Answer from the drawing. Dimensions are ordinates in mm from the lowest x, y and z of the part. Give positions to 0.01 mm unless a question says otherwise; leave off trailing zeros. Write each loop counter-clockwise with the first axis right and the second up, starting at its lowest first coordinate (ties: lowest second). Pieces come first, ordered by that corner, then holes. Notation, with made-up numbers: (59.25, 75) -> (92.25, 75) arc R20 cw to (92.25, 111) -> close; hole circle Ø3 at (74, 74.5). An arc over 180 degrees is marked (long way). Write item = value, one per line.
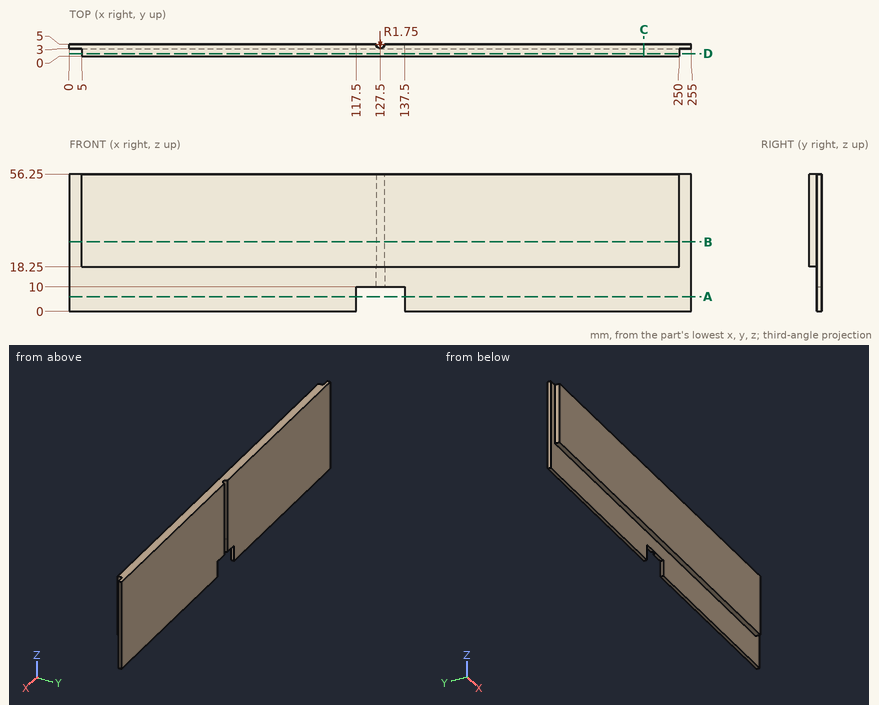
(1) The part is cut by section A-A on z = 6. Determine the outline of the cut face in (x, y).
Checks:
outline = (0, 3) -> (117.5, 3) -> (117.5, 5) -> (0, 5) -> close; (137.5, 3) -> (255, 3) -> (255, 5) -> (137.5, 5) -> close
(2) Consider L1, parallel to X at y = 4.1, z = 9.5; L2, parallel to X at y = 0.4, z = 18.5; L3, parallel to Y at x = 104, z = 18. Determine where each line is inside the solid, lowest interval first.
Checks:
L1 = 0 to 117.5, 137.5 to 255
L2 = 5 to 250
L3 = 3 to 5
(3) The part is cut by section B-B on z = 28.5. Determine the outline of the cut face in (x, y), plus the area to 3 significant figures.
Checks:
outline = (0, 3) -> (5, 3) -> (5, 0) -> (250, 0) -> (250, 3) -> (255, 3) -> (255, 5) -> (129.25, 5) arc R1.75 cw to (125.75, 5) -> (0, 5) -> close
area = 1,240 mm²
(4) The part is cut by section C-C on x = 235.5. Determine the outline of the cut face in (y, z), plus the area to 4 significant figures.
Checks:
outline = (0, 18.25) -> (3, 18.25) -> (3, 0) -> (5, 0) -> (5, 56.25) -> (0, 56.25) -> close
area = 226.5 mm²
(5) Given P1, Ø2, axis at x = 130.5, y = 4, coming from the -Z side; P2, Ø1.6, axis at y = 4, z = 2.5, coming from the -X side; P3, Ø0.9, axis at y = 2, z = 29, coming from the -X side; P4, Ø2, axis at x = 26.5, y = 1, coming from the -Z side, each flat-ended and moving along its own axis, determine where each tip first touches the part or whether it passes through.
Checks:
P1 = 10
P2 = 0
P3 = 5
P4 = 18.25
(6) The part is cut by section D-D on y = 1.05. Determine the outline of the cut face in (x, z).
Checks:
outline = (5, 18.25) -> (250, 18.25) -> (250, 56.25) -> (5, 56.25) -> close
